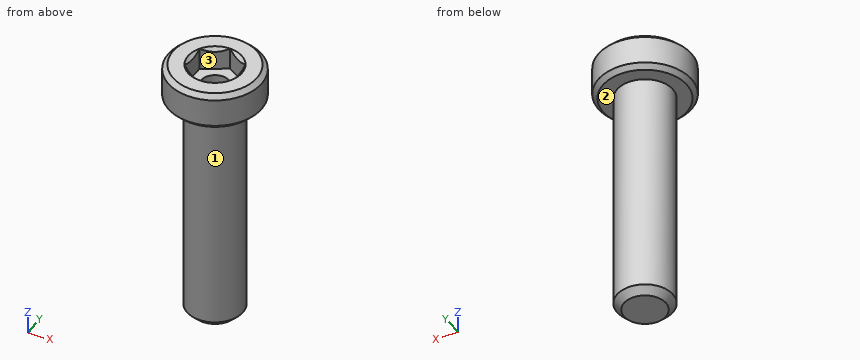
```python
from build123d import *

# Parameters (mm, degrees)
SKETCH1_W              = 25
SKETCH1_H              = 3
CHAMFER1_SIZE          = 0.5
CUT_EXTRUDE1_DEPTH     = 2.38
SPLIT1_SURFACE_1_BACK  = 33.265
SPLIT1_SURFACE_1_DEPTH = 66.53
SPLIT1_SURFACE_2_BACK  = 33.265
SPLIT1_SURFACE_2_DEPTH = 66.53
CHAMFER2_SIZE          = 0.75


with BuildPart() as part:
    # Sketch1 → Revolve1 (revolve)
    with BuildSketch(Plane.ZY, mode=Mode.PRIVATE) as revolve1_sk:
        Polygon((25, 3), (25, 0), (29, 0), (29, 5), (25, 5), align=None)
        with Locations((12.5, 1.5)):
            Rectangle(SKETCH1_W, SKETCH1_H)
    revolve(revolve1_sk.sketch.rotate(Axis((0, 0, 25), (0, 0, 1)), 90), axis=Axis((0, 0, 25), (0, 0, 1)))

    # Chamfer1
    chamfer1_edges = [part.edges().sort_by_distance(p)[0] for p in [
        (5, 0, 29),
        (5, 0, 25),
    ]]
    chamfer(chamfer1_edges, length=CHAMFER1_SIZE)

    # Sketch2 → Cut-Extrude1 (cut)
    with BuildSketch(Plane.XY.offset(29)):
        Polygon((0, 2.886751346), (-2.5, 1.443375673), (-2.5, -1.443375673), (0, -2.886751346), (2.5, -1.443375673), (2.5, 1.443375673), align=None)
    extrude(amount=-CUT_EXTRUDE1_DEPTH, mode=Mode.SUBTRACT)

    # Sketch3 → Cut-Revolve1 (revolve, cut)
    with BuildSketch(Plane(origin=(0, 0, 11.32), x_dir=(0, 0, 1), z_dir=(-1, 0, 0)), mode=Mode.PRIVATE) as cut_revolve1_sk:
        Polygon((13.619461487, 1.5), (12.92, 0), (15.3, 0), (15.3, 1.5), align=None)
    revolve(cut_revolve1_sk.sketch.rotate(Axis((0, 0, 26.62), (0, 0, -1)), 180), axis=Axis((0, 0, 26.62), (0, 0, -1)), mode=Mode.SUBTRACT)

    # Cut-Extrude2 cone 1 section (on through the dimple's axis) → Cut-Extrude2 (revolve, cut)
    with BuildSketch(Plane(origin=(0, 0, 29), x_dir=(0, -1, 0), z_dir=(1, 0, 0))):
        Polygon((0, 0), (2.886751346, 0), (0, 2.886751346), align=None)
    revolve(axis=Axis((0, 0, 29), (0, 0, -1)), mode=Mode.SUBTRACT)


with BuildPart() as body_2:
    # Split1: the piece behind the surface
    add(part.part)
    # Split1 surface: a surface, the sketch's curves swept straight by 66.53 mm
    with BuildLine(Plane(origin=(0, 0, 0), x_dir=(0, 0, -1), z_dir=(1, 0, 0)).offset(-SPLIT1_SURFACE_1_BACK), mode=Mode.PRIVATE) as split1_surface_1_path:
        Line((-19.5, 3), (-19.5, -3))
    split1_surface_1 = Shell.extrude(split1_surface_1_path.wire(), (1 * SPLIT1_SURFACE_1_DEPTH, 0 * SPLIT1_SURFACE_1_DEPTH, 0 * SPLIT1_SURFACE_1_DEPTH))
    split(bisect_by=split1_surface_1, keep=Keep.BOTTOM)


with BuildPart() as part_1:
    add(part.part)

    # Split1: split by a surface, the side it looks to stays
    # Split1 surface: a surface, the sketch's curves swept straight by 66.53 mm
    with BuildLine(Plane(origin=(0, 0, 0), x_dir=(0, 0, -1), z_dir=(1, 0, 0)).offset(-SPLIT1_SURFACE_2_BACK), mode=Mode.PRIVATE) as split1_surface_2_path:
        Line((-19.5, 3), (-19.5, -3))
    split1_surface_2 = Shell.extrude(split1_surface_2_path.wire(), (1 * SPLIT1_SURFACE_2_DEPTH, 0 * SPLIT1_SURFACE_2_DEPTH, 0 * SPLIT1_SURFACE_2_DEPTH))
    split(bisect_by=split1_surface_2, keep=Keep.TOP)

    # Chamfer2
    chamfer2_edges = [part_1.edges().sort_by_distance(p)[0] for p in [
        (3, 0, 0),
    ]]
    chamfer(chamfer2_edges, length=CHAMFER2_SIZE)


with BuildPart() as body_2_1:
    add(body_2.part)

    # Combine1: union part
    add(part_1.part)


solid = body_2_1.part
```
Read the model definition and answer for the solid it produces. Units are mm, in the model's axes. Face numbers are marked on the shaded views. Give positions to 0.01 mm unless a question says otherwise; leave off trailing zeros. Write each loop counter-clockwise with the first axis right and the second up, starting at its lowest first coordinate (ties: lowest second). Pieces come first, ordered by that corner, then holes. Notation, with made-up numbers: M 41,-12 L 50,-12 A8 ccw 50,1 Z; hole C -28,-8 d6. An arc over 180 degrees is marked long. Put each result on its own line as item: value. Start each with the question number.
1. The part is cut by section A-A, the plane z = 17.75. Give the vertices of the cut face in (x, y).
2. For a pull along Y with two mould halves and no side action, classify the marked faces 1, 2 and 3 as released by +Y, released by -Y, zero draft, split by the parting line, or undercut.
3. Each of these flat-tipped pins is pushed along its axis until it touches: pin 1 Ø6 at (x, z) = (-0.5, 6) entering from +Y; pin 2 Ø6 at (y, z) = (1, 20.5) entering from +X; pin 3 Ø3 at (y, z) = (3.5, 18) entering from -X. Where does it stop, or does it pass through?
4. Consider line 1 along Z through (x, y) = (-3.75, -2); line 2 along Z through (x, y) = (1.25, -1.25); line 3 along Y through (x, z) = (1.75, 27). Determine where each line is inside the solid, lowest interval first.
Final values:
1. outline: C 0,0 d6
2. face 1: split by the parting line
2. face 2: zero draft
2. face 3: undercut
3. pin 1: stops at y = 3
3. pin 2: stops at x = 3
3. pin 3: stops at x = -2.24
4. line 1: z = 25 to 29
4. line 2: z = 0 to 26.62
4. line 3: y = -4.68 to -1.88, 1.88 to 4.68
